Can you work these out from the drawing? Everything is in mm from the part's minimum corner. Round coordinates to 2 decimals unless told otherwise and drop trailing zeros. Loops run counter-clockwise (first coordinate to the right, second up) from the corner with the lowest first, then second, coordinate; pieces in that order, holes last. Notation, with made-up numbers: (59.25, -33) - (100.25, -33) arc R19 cw to (100.25, -8) - close; hole circle Ø11 at (57.5, 85). An arc over 180 degrees is marked (long way). Answer as CSV lines item,"result". Start each with the question number.
1) Suppose I cut it at A-A, the plane z = 2. Write out the boundary of the cut face in (x, y), then the cut area to 3 significant figures.
2) Suppose I cut it at B-B, the plane y = 61.5. Write out the boundary of the cut face in (x, z).
3) I'm going to push a flat-ended pin straight in: pin 1 Ø5 at (x, y) = (40.5, 66.5) entering from +Z. Where does the tip first touch, or does it pass through?
4) Suppose I cut it at C-C, the plane x = 56. Write out the boundary of the cut face in (y, z).
5) Please list where these lines run through material, in increasing order: line 1 along X through (y, z) = (61.5, 2.9); line 2 along Y through (x, z) = (28.5, 2.15).
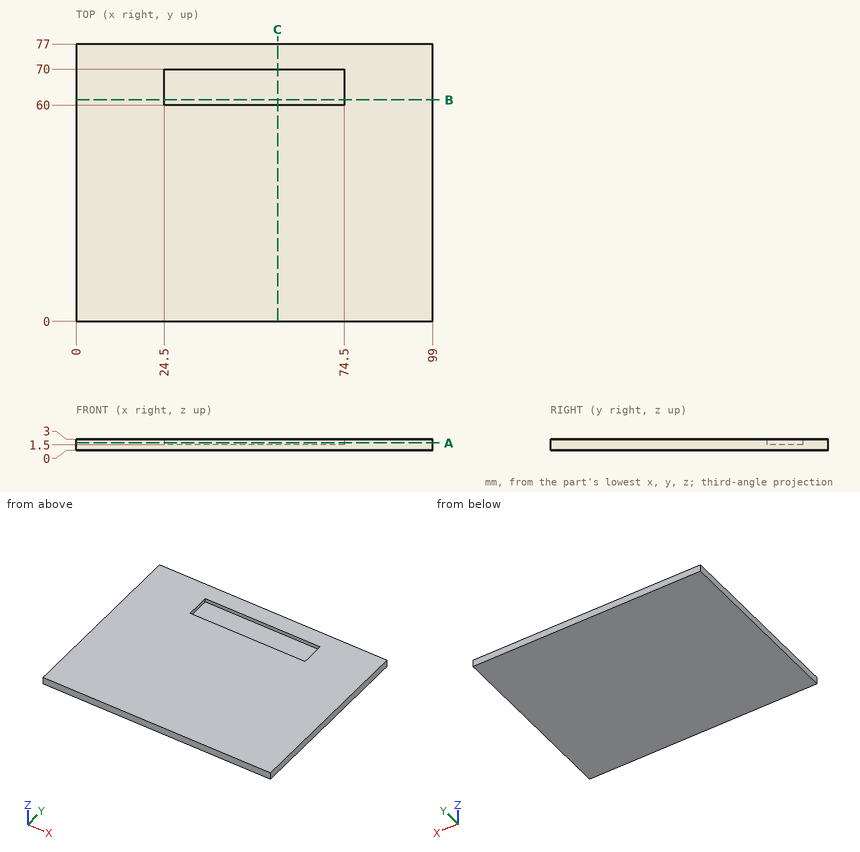
Filled sheet:
1,outline,"(0, 0) - (99, 0) - (99, 77) - (0, 77) - close; hole (24.5, 60) - (74.5, 60) - (74.5, 70) - (24.5, 70) - close"
1,area,"7,120 mm²"
2,outline,"(0, 0) - (99, 0) - (99, 3) - (74.5, 3) - (74.5, 1.5) - (24.5, 1.5) - (24.5, 3) - (0, 3) - close"
3,pin 1,"z = 1.5"
4,outline,"(0, 0) - (77, 0) - (77, 3) - (70, 3) - (70, 1.5) - (60, 1.5) - (60, 3) - (0, 3) - close"
5,line 1,"0 to 24.5, 74.5 to 99"
5,line 2,"0 to 60, 70 to 77"
